from build123d import *

# Parameters (mm, degrees)
SKETCH1_R           = 47.625
BOSS_EXTRUDE1_DEPTH = 21
SKETCH2_R           = 42.625
CUT_EXTRUDE1_DEPTH  = 10
SKETCH3_W           = 70
SKETCH3_H           = 40
BOSS_EXTRUDE2_DEPTH = 15
SKETCH4_R           = 7.5
CUT_EXTRUDE2_DEPTH  = 86.336283315
SKETCH5_R           = 2.6
CUT_EXTRUDE3_DEPTH  = 77.36937377
SKETCH6_R           = 11.5
CUT_EXTRUDE4_DEPTH  = 16.5


with BuildPart() as part:
    # Sketch1 → Boss-Extrude1 (new body)
    with BuildSketch(Plane.XY):
        with Locations(Location((0, 0, 0), (0, 0, 180))):
            Circle(SKETCH1_R)
    extrude(amount=BOSS_EXTRUDE1_DEPTH)

    # Sketch2 → Cut-Extrude1 (cut)
    with BuildSketch(Plane.XY.offset(21)):
        Circle(SKETCH2_R)
    extrude(amount=-CUT_EXTRUDE1_DEPTH, mode=Mode.SUBTRACT)

    # Sketch3 → Boss-Extrude2 (add)
    with BuildSketch(Plane(origin=(0, 0, 0), x_dir=(-1, 0, 0), z_dir=(0, 0, -1))):
        Rectangle(SKETCH3_W, SKETCH3_H)
    extrude(amount=BOSS_EXTRUDE2_DEPTH)

    # Sketch4 → Cut-Extrude2 (cut, through all)
    with BuildSketch(Plane(origin=(0, 20, 0), x_dir=(-1, 0, 0), z_dir=(0, 1, 0))):
        with Locations((-20, -15)):
            Circle(SKETCH4_R)
        with Locations((20, -15)):
            Circle(SKETCH4_R)
    extrude(amount=-CUT_EXTRUDE2_DEPTH, mode=Mode.SUBTRACT)

    # Sketch5 → Cut-Extrude3 (cut, through all)
    with BuildSketch(Plane(origin=(0, 0, -15), x_dir=(-1, 0, 0), z_dir=(0, 0, -1))):
        Circle(SKETCH5_R)
    extrude(amount=-CUT_EXTRUDE3_DEPTH, mode=Mode.SUBTRACT)

    # Sketch6 → Cut-Extrude4 (cut, symmetric)
    with BuildSketch(Plane(origin=(0, 0, 0), x_dir=(1, 0, 0), z_dir=(0, 1, 0))):
        with Locations((-20, 15)):
            Circle(SKETCH6_R)
        with Locations((20, 15)):
            Circle(SKETCH6_R)
    extrude(amount=CUT_EXTRUDE4_DEPTH, both=True, mode=Mode.SUBTRACT)


solid = part.part
Can you work these out from the model? Positions are in its coordinate system, mm. A direction names the side the tool comes from. Round coordinates to 2 decimals unless told otherwise and drop trailing zeros. Write each loop counter-clockwise with the first axis right and the second up, starting at its lowest first coordinate (ties: lowest second). Pieces come first, ordered by that corner, then holes. Notation, with made-up numbers: M -1,30.5 L 36,30.5 A6 cw 36,39.5 Z; hole C 57.5,85 d4. An arc over 180 degrees is marked long. Use CSV: the item, a comma, the result in double quotes.
(1) I need wall thicknesses on line 1 along Y through (x, z) = (0, 16) (3 decimals); line 2 along X through (y, z) = (15.5, -6); line 3 along Y through (x, z) = (0, -3). Which ranges of each line are inside material? Lowest first, please.
Check values:
line 1,"-47.625 to -42.625, 42.625 to 47.625"
line 2,"-35 to -27.16, -12.84 to 12.84, 27.16 to 35"
line 3,"-20 to -2.6, 2.6 to 20"
(2) Imagine slicing it at C-C (z = 18). Write out the boundary of the cut face in (x, y) (3 decimals), plus the area to 3 significant figures.
Check values:
outline,"C 0,0 d95.25; hole C 0,0 d85.25"
area,"1,420 mm^2"
(3) On a 3-axis mill with a long thin cutter (end or side, diameter ignored), from which of +Z, -Z, +X, -X, +Y, -Y can I reach the whole of each face in a straight line? I mean faces 1 (the flat face through (-20, -16.5, -7)), 2 (the flat face through (0, -20, -6)), 3 (the cylindrical face through (0.338, 2.578, -2.182)). Say none if no direction works.
Check values:
face 1,"-Z"
face 2,"-Z, +X, -X, -Y"
face 3,"+Z, -Z"
(4) We'd pull the mould along X, two halves only. Please class faces 4 (the flat face through (0, 20, -6)), 5 (the flat face through (-1, -9, 11)), 6 (the flat face through (35, 0, -7)): +X half, -X half, draft (parallel to the pull), parting line (faces both ways), or undercut.
Check values:
face 4,"draft"
face 5,"undercut"
face 6,"+X half"
(5) Imagine slicing it at B-B (z = -5.5). Write out the boundary of the cut face in (x, y), plus the area to 3 significant figures.
Check values:
outline,"M -35,-20 L 35,-20 L 35,20 L -35,20 Z; hole M -26.48,-16.5 L -13.52,-16.5 L -13.52,16.5 L -26.48,16.5 Z; hole C 0,0 d5.2; hole M 13.52,-16.5 L 26.48,-16.5 L 26.48,16.5 L 13.52,16.5 Z"
area,"1,920 mm^2"
(6) Imagine slicing it at D-D (y = -37.5). Write out the boundary of the cut face in (x, z), plus the area to 3 significant figures.
Check values:
outline,"M -29.36,0 L 29.36,0 L 29.36,21 L 20.26,21 L 20.26,11 L -20.26,11 L -20.26,21 L -29.36,21 Z"
area,"828 mm^2"
(7) Imagine slicing it at A-A (x = 0). Write out the boundary of the cut face in (y, z) (3 decimals), plus the area to 3 significant figures.
Check values:
outline,"M -47.625,0 L -20,0 L -20,-15 L -2.6,-15 L -2.6,11 L -42.625,11 L -42.625,21 L -47.625,21 Z; M 2.6,-15 L 20,-15 L 20,0 L 47.625,0 L 47.625,21 L 42.625,21 L 42.625,11 L 2.6,11 Z"
area,"1,610 mm^2"
(8) I'm going to push flat-ended pins straight in: pin 1 (10 mm diameter, centred on y = -6, z = -9, fed in from -X); pin 2 (7.5 mm diameter, centred on y = -2.5, z = -10, fed in from +X); pin 3 (4.5 mm diameter, centred on x = 17.5, z = -8.5, fed in from -Y); pin 4 (6 mm diameter, centred on x = -23, z = -12, fed in from +Y). Where does each tip first touch, or does it pass through?
Check values:
pin 1,"x = -35"
pin 2,"x = 35"
pin 3,"y = -20"
pin 4,"through"
